For this review, take the finished solid that the model builds, in its own axes (mm). A direction names the side the tool comes from. Round coordinates to 2 decimals unless told otherwise and drop trailing zeros. Order: outer loops, then holes, each group sorted by start corner. A loop starts at its lowest first (then second) coordinate and runs counter-clockwise, first axis right, second up. Notation, with made-up numbers: M 76,62 L 123,62 A22 cw 123,90 Z; hole C -6.75,50 d4. An arc over 180 degrees is marked long. Use a Markdown table: item, result.
Autodesk Inventor part; units mm, degrees
ref_plane "YZ Plane" through (0, 0, 0) normal (1, 0, 0) x (0, 1, 0)
ref_plane "XZ Plane" through (0, 0, 0) normal (0, 1, 0) x (-1, 0, 0)
ref_plane "XY Plane" through (0, 0, 0) normal (0, 0, 1) x (1, 0, 0)
sketch "スケッチ1" plane through (0, 0, 0) normal (0, 1, 0) x (-1, 0, 0)
  line L0 (-4, -9) -> (4, -9)
  line L1 (9, -4) -> (9, 4)
  line L2 (4, 9) -> (-4, 9)
  line L3 (-9, 4) -> (-9, -4)
  arc A0 (9, 4) -> (4, 9) centre (4, 4) ccw
  arc A1 (-4, 9) -> (-9, 4) centre (-4, 4) ccw
  arc A2 (-9, -4) -> (-4, -9) centre (-4, -4) ccw
  arc A3 (4, -9) -> (9, -4) centre (4, -4) ccw
  point P0 (0, 0)
  point P1 (9, 0)
  point P2 (0, -9)
  point P3 (9, 4)
  point P4 (9, -4)
  point P5 (4, 9)
  point P6 (-4, 9)
  point P7 (-9, -4)
  point P8 (4, -9)
  dimension "d0" = 5
extrude "押し出し1" add sketch "スケッチ1" along normal blind 10
sketch "スケッチ2" plane through (0, 10, 0) normal (0, 1, 0) x (1, 0, 0)
  circle A0 centre (0, 0) radius 8.7
  dimension "d3" = 17.4
extrude "押し出し2" add sketch "スケッチ2" along normal blind 200
sketch "スケッチ3" plane through (0, 210, 0) normal (0, 1, 0) x (1, 0, 0)
  point P0 (0, 0)
sketch "スケッチ4" plane through (0, 210, 0) normal (0, 1, 0) x (1, 0, 0)
  line L0 (-4, 9) -> (4, 9)
  line L1 (4, 9) -> (-4, 9)
  line L2 (9, 4) -> (9, -4)
  line L3 (4, -9) -> (-4, -9)
  line L4 (-9, -4) -> (-9, 4)
  arc A0 (-9, -4) -> (-4, -9) centre (-4, -4) ccw
  arc A1 (-4, 9) -> (-9, 4) centre (-4, 4) ccw
  arc A2 (9, 4) -> (4, 9) centre (4, 4) ccw
  arc A3 (4, -9) -> (9, -4) centre (4, -4) ccw
  point P0 (0, 0)
  point P1 (-9, 9)
  point P2 (9, 9)
  dimension "d6" = 18
  dimension "d7" = 5
extrude "押し出し3" add sketch "スケッチ4" along normal blind 12.4
sketch "スケッチ5" plane through (0, 222.4, 0) normal (0, 1, 0) x (1, 0, 0)
  circle A0 centre (0, 0) radius 5
  dimension "d10" = 10
extrude "押し出し4" add sketch "スケッチ5" along normal blind 8
sketch "スケッチ6" plane through (0, 230.4, 0) normal (0, 1, 0) x (1, 0, 0)
  circle A0 centre (0, 0) radius 2.5
  dimension "d13" = 5
extrude "押し出し5" cut sketch "スケッチ6" against normal blind 180
sketch "スケッチ7" plane through (9, 0, 4) normal (1, 0, 0) x (0, 0, -1)
  line L0 (4, 0) -> (4, 10)
  line L1 (0, 10) -> (8, 10)
  circle A0 centre (4, 5) radius 2
  dimension "d16" = 4
extrude "押し出し6" cut sketch "スケッチ7" against normal blind 11.6
sketch "スケッチ8" plane through (9, 210, 4) normal (1, 0, 0) x (0, 0, -1)
  line L0 (0, 0) -> (8, 0)
  line L1 (4, 0) -> (4, 12.4)
  line L2 (-1, 12.4) -> (9, 12.4)
  circle A0 centre (4, 4.5) radius 2
  point P0 (4, -210)
  dimension "d19" = 4.5
  dimension "d20" = 4
extrude "押し出し7" cut sketch "スケッチ8" against normal blind 6.9
properties part number "SMC_CJ2B16-175(本体)"
Q1. Add section B-B (y = 5). Write out the cut boundary in (x, z), then the cut area to 3 significant figures.
Determined:
| item | result |
|---|---|
| outline | M -9,-4 A5 ccw -4,-9 L 4,-9 A5 ccw 9,-4 L 9,-2 L -2.6,-2 L -2.6,2 L 9,2 L 9,4 A5 ccw 4,9 L -4,9 A5 ccw -9,4 Z |
| area | 256 mm^2 |
Q2. Add section A-A (x = 0). Write out the cut boundary in (y, z).
Determined:
| item | result |
|---|---|
| outline | M 0,-9 L 10,-9 L 10,-8.7 L 210,-8.7 L 210,-9 L 222.4,-9 L 222.4,-5 L 230.4,-5 L 230.4,-2.5 L 50.4,-2.5 L 50.4,2.5 L 230.4,2.5 L 230.4,5 L 222.4,5 L 222.4,9 L 210,9 L 210,8.7 L 10,8.7 L 10,9 L 0,9 Z; hole C 5,0 d4 |
Q3. Draft analysis for pull direction Y (two halves, no side actions). For faces 4 (the flat face through (-4, 222.4, 4)), 5 (the cylindrical face through (-1.08, 226.34, -4.88)), 6 (the cylindrical face through (-1.886, 108.6, -8.493)), state which applies: pulls with the +Y half, pulls with the -Y half, needs draft (parallel to the pull), parting line crosses it, or undercut.
Determined:
| item | result |
|---|---|
| face 4 | pulls with the +Y half |
| face 5 | needs draft |
| face 6 | undercut |
Q4. Wall thickness on line 1 along Y through (x, z) = (5.5, 0); line 2 along Y through (x, z) = (2.75, 0); line 3 along Z through (x, y) = (-0.5, 5): over which ranges is each line inside the solid? List them lowest first. Write a range as [from, to].
Determined:
| item | result |
|---|---|
| line 1 | y = [0, 3], [7, 212.5], [216.5, 222.4] |
| line 2 | y = [0, 3], [7, 212.5], [216.5, 230.4] |
| line 3 | z = [-9, -2], [2, 9] |
Q5. Add section C-C (y = 90). Write out the cut boundary in (x, z).
Determined:
| item | result |
|---|---|
| outline | C 0,0 d17.4; hole C 0,0 d5 |
Q6. Clearance check with flat-ended pins moving along their axes: pin 1 (3 mm diameter, centred on x = -3, y = 177.5, fed in from -Z); pin 2 (6 mm diameter, centred on x = -6.5, y = 73.5, fed in from -Z); pin 3 (6 mm diameter, centred on x = -0.5, y = 88.5, fed in from +Z); pin 4 (4.5 mm diameter, centred on y = 5, z = 0, fed in from +X). State where each tip first meets the part, or that it passes through.
Determined:
| item | result |
|---|---|
| pin 1 | stops at z = -8.57 |
| pin 2 | stops at z = -7.96 |
| pin 3 | stops at z = 8.7 |
| pin 4 | stops at x = 9 |
Q7. Machinability: for faces 1 (the flat face through (0, 50.4, 0)), 2 (the cylindrical face through (3, 7, 0)), 3 (the flat face through (-6, 210, -7)), which of the approach directions +Z, -Z, +X, -X, +Y, -Y give a long, thin tool a straight path to every point of the face, cutting with its end or side? Answer none if there is none.
Determined:
| item | result |
|---|---|
| face 1 | +Y |
| face 2 | +X |
| face 3 | none |
